Here's the drawing with two shaded views (mm, measured from the low corner). I have some questions. A direction names the side the tool comes from. Coordinates: 2 decimals unless noted, no trailing zeros. Write each loop counter-clockwise with the first axis right and the second up, starting at its lowest first coordinate (ties: lowest second). Pieces come first, ordered by that corner, then holes.
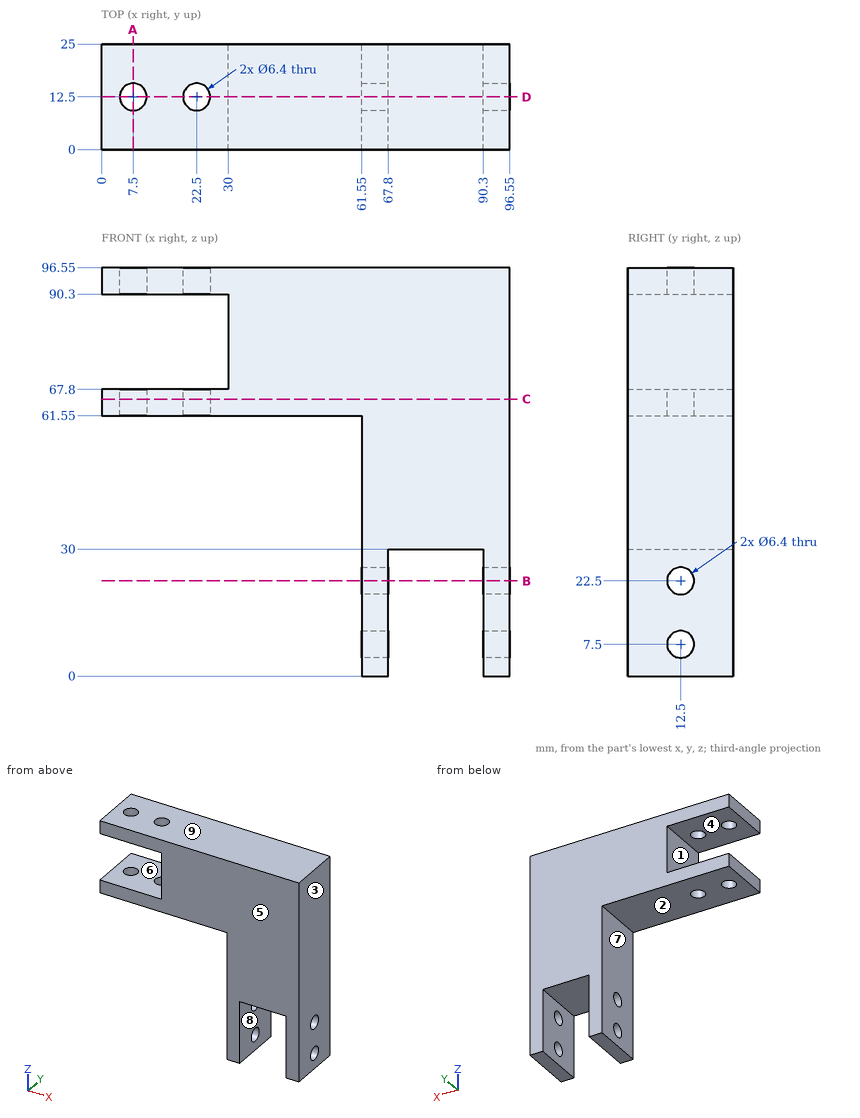
1. If we section it at A-A, the plane x = 7.5: List the corners of the cut face in (y, z) for me, plus the area to 4 significant figures.
2. If we section it at C-C, the plane z = 65.5: List the corners of the cut face in (x, y) for me, plus the area to 3 significant figures.
3. Which directions (+Z, -Z, +X, -X, +Y, -Y) give clear straight access to the entire face, cutting with the end or side of a thin tool? Please do the marked faces 5, 6, 7, 8 and 9.
4. We'd pull the mould along Z, two halves only. Please class the marked faces 1, 2, 3 and 4: released by +Z, released by -Z, zero draft, split by the parting line, or undercut.
5. I'm going to push flat-ended pins straight in: P1, Ø1.5, axis at y = 15.5, z = 22.5, coming from the -X side; P2, Ø12.5, axis at x = 15, y = 14, coming from the -Z side; P3, Ø7, axis at x = 80.5, y = 13, coming from the -Z side. Where does each tip first touch, or does it pass through?
6. If we section it at D-D, the plane y = 12.5: Count the separate pieces of the cut face and the enclosed holes in it, plus the area to 3 significant figures.
7. If we section it at B-B, the plane z = 22.5: List the corners of the cut face in (x, y) for me.
8. If I drill on L1, parallel to Z at x = 29, y = 19.75; L2, parallel to Z at x = 73, y = 8.5, over which ranges is the centre line in solid material (lowest first)?
Answers:
1. outline: (0, 61.55) - (9.3, 61.55) - (9.3, 67.8) - (0, 67.8) - close; (0, 90.3) - (9.3, 90.3) - (9.3, 96.55) - (0, 96.55) - close; (15.7, 61.55) - (25, 61.55) - (25, 67.8) - (15.7, 67.8) - close; (15.7, 90.3) - (25, 90.3) - (25, 96.55) - (15.7, 96.55) - close
1. area: 232.5 mm2
2. outline: (0, 0) - (96.55, 0) - (96.55, 25) - (0, 25) - close; hole circle Ø6.4 at (7.5, 12.5); hole circle Ø6.4 at (22.5, 12.5)
2. area: 2,350 mm2
3. face 5: +Z, -Z, +X, -X, -Y
3. face 6: -X, +Y, -Y
3. face 7: -Z, -X, +Y, -Y
3. face 8: -Z, +Y, -Y
3. face 9: +Z, +X, -X, +Y, -Y
4. face 1: undercut
4. face 2: released by -Z
4. face 3: zero draft
4. face 4: undercut
5. P1: stops at x = 61.55
5. P2: stops at z = 61.55
5. P3: stops at z = 30
6. separate pieces: 9
6. enclosed holes: 0
6. area: 3,860 mm2
7. outline: (61.55, 0) - (67.8, 0) - (67.8, 9.3) - (61.55, 9.3) - close; (61.55, 15.7) - (67.8, 15.7) - (67.8, 25) - (61.55, 25) - close; (90.3, 0) - (96.55, 0) - (96.55, 9.3) - (90.3, 9.3) - close; (90.3, 15.7) - (96.55, 15.7) - (96.55, 25) - (90.3, 25) - close
8. L1: z = 61.55 to 67.8, 90.3 to 96.55
8. L2: z = 30 to 96.55
